Design review of the part built by this model. Coordinates are the model's own, in mm. A direction names the side the tool comes from. Give positions to 0.01 mm unless a question says otherwise; leave off trailing zeros. Loops run counter-clockwise (first coordinate to the right, second up) from the corner with the lowest first, then second, coordinate; pieces in that order, holes last. Notation, with made-up numbers: (-25, 46) -> (24, 46) arc R30 ccw to (24, 68) -> close; hole circle Ø7 at (46.25, -37). An arc over 180 degrees is marked (long way). Use a Markdown table: item, result. Add a question column.
1. For pin 1 Ø2.5 at (x, y) = (17.5, 12.5) entering from -Z; pin 2 Ø1.5 at (x, z) = (15.5, -5) entering from +Y; pin 3 Ø7.5 at (x, y) = (13.5, 16.5) entering from -Z; pin 4 Ø10 at (y, z) = (2.5, -2.5) entering from -X, all flat-tipped, find the tip position at first contact; note any pin that passes through.
2. To check wall thickness, follow line 1 (Y direction, x = 12.5, z = 0.7); line 2 (Y direction, x = 9.25, z = -21.25); line 3 (Z direction, x = 16, y = 3.75). State the ranges of each line that lie inside material, in increasing order.
3. Add section A-A (y = 12.5). State the section outline as (x, z) points, and give its area (3 significant figures).
4. Draft analysis for pull direction Y (two halves, no side actions). For faces 1 (the flat face through (12.5, 25, 0.5)), 2 (the cylindrical face through (22.15, -0.51, -20.99)), 3 (the cylindrical face through (6.3, 11.6, 0.5)), state which applies: pulls with the +Y half, pulls with the -Y half, needs draft (parallel to the pull), parting line crosses it, or undercut.
5. Add section D-D (y = 7.75). State the section outline as (x, z) points.
6. Add section B-B (x = 12.5). State the section outline as (y, z) points, and give its area (3 significant figures).
7. Add section C-C (z = -12.5). State the section outline as (x, y) points.
8. For faces 4 (the cylindrical face through (2.85, -0.51, -20.99)), 5 (the flat face through (10, 10, 0)), list the 3-axis set-ups (+Z, -Z, +X, -X, +Y, -Y) from which the entire face can be reached by the end or side of a thin tool; tool diameter is ignored.
```python
from build123d import *

# Parameters (mm, degrees)
SKETCH1_W      = 25
SKETCH1_H      = 25
SKETCH1_R      = 3.05
SKETCH1_R_2    = 1.5
EXTRUDE1_DEPTH = 1
SKETCH2_W      = 25
SKETCH2_H      = 25
EXTRUDE2_DEPTH = 1
FILLET1_R      = 10


with BuildPart() as part:
    # Sketch1 → Extrude1 (new body)
    with BuildSketch(Plane.XY):
        with Locations((12.5, 12.5)):
            Rectangle(SKETCH1_W, SKETCH1_H)
        with Locations((12.5, 12.5)):
            Circle(SKETCH1_R, mode=Mode.SUBTRACT)
        with Locations((17.5, 12.5)):
            Circle(SKETCH1_R_2, mode=Mode.SUBTRACT)
        with Locations((7.5, 12.5)):
            Circle(SKETCH1_R_2, mode=Mode.SUBTRACT)
    extrude(amount=EXTRUDE1_DEPTH)

    # Sketch2 → Extrude2 (add)
    with BuildSketch(Plane.XZ):
        with Locations((12.5, -11.5)):
            Rectangle(SKETCH2_W, SKETCH2_H)
    extrude(amount=EXTRUDE2_DEPTH)

    # Fillet1
    fillet1_edges = [part.edges().sort_by_distance(p)[0] for p in [
        (0, -0.5, -24),
        (25, -0.5, -24),
        (0, 25, 0.5),
        (25, 25, 0.5),
    ]]
    fillet(fillet1_edges, radius=FILLET1_R)


solid = part.part
```
Taken from the geometry:
| question | item | result |
|---|---|---|
| 1 | pin 1 | passes through |
| 1 | pin 2 | stops at y = 0 |
| 1 | pin 3 | stops at z = 0 |
| 1 | pin 4 | stops at x = 0 |
| 2 | line 1 | y = -1 to 9.45, 15.55 to 25 |
| 2 | line 2 | y = -1 to 0 |
| 2 | line 3 | z = 0 to 1 |
| 3 | outline | (0, 0) -> (6, 0) -> (6, 1) -> (0, 1) -> close; (9, 0) -> (9.45, 0) -> (9.45, 1) -> (9, 1) -> close; (15.55, 0) -> (16, 0) -> (16, 1) -> (15.55, 1) -> close; (19, 0) -> (25, 0) -> (25, 1) -> (19, 1) -> close |
| 3 | area | 12.9 mm^2 |
| 4 | face 1 | pulls with the +Y half |
| 4 | face 2 | needs draft |
| 4 | face 3 | undercut |
| 5 | outline | (0, 0) -> (25, 0) -> (25, 1) -> (0, 1) -> close |
| 6 | outline | (-1, -24) -> (0, -24) -> (0, 0) -> (9.45, 0) -> (9.45, 1) -> (-1, 1) -> close; (15.55, 0) -> (25, 0) -> (25, 1) -> (15.55, 1) -> close |
| 6 | area | 43.9 mm^2 |
| 7 | outline | (0, -1) -> (25, -1) -> (25, 0) -> (0, 0) -> close |
| 8 | face 4 | -Z, -X, +Y, -Y |
| 8 | face 5 | -Z, +X, -X, +Y |
